Verification items for the finished model (mm, model axes). Give positions to 0.01 mm unless a question says otherwise; leave off trailing zeros. One line per item, written item: value. Start each with the question number.
1. Mould release check, pull along Y, two halves, no side actions. Record for faces 1 (the cylindrical face through (0, 21, 4)), 2 (the cylindrical face through (-36.244, 0.275, 4.437)), 3 (the flat face through (-10, -8, 0)): pulls with the +Y half, pulls with the -Y half, needs draft (parallel to the pull), parting line crosses it, or undercut.
2. Gauge pin test, flat ends, axial feed: pin 1 (5 mm diameter, centred on x = -1.5, z = 2, fed in from +Y); pin 2 (2 mm diameter, centred on y = -7.5, z = 6.5, fed in from +X); pin 3 (4 mm diameter, centred on y = -14.5, z = 3.5, fed in from +X); pin 4 (11 mm diameter, centred on x = -30, y = 0, fed in from +Z). Record the tip position at first contact, or that the pin passes through.
3. Sectioned sample at A-A (y = 2). Count the separate pieces of the cut face and the enclosed holes in it, plus the area to 3 significant figures.
4. Scan lines: L1, parallel to Y at x = 0, z = 6; L2, parallel to Y at x = -30, z = 3.5; L3, parallel to X at y = -3.5, z = 6.75. Record each from-to range of solid material in increasing order. Write a range as [from, to].
from build123d import *

# Parameters (mm, degrees)
F0_R     = 6.25
F0_R_2   = 11
F1_DEPTH = 9
F2_R     = 5
F3_R     = 3
F4_R     = 3


with BuildPart() as f1:
    # F0 (on Top) → F1 (new body)
    with BuildSketch(Plane.XY):
        with BuildLine():
            ThreePointArc((18.965625, 9.0169323142), (20.4850936659, 4.6217894262), (21, 0))
            ThreePointArc((21, 0), (20.4850936659, -4.6217894262), (18.965625, -9.0169323142))
            ThreePointArc((18.965625, -9.0169323142), (34.7865779138, -13.4220405258), (44.25, 0))
            ThreePointArc((44.25, 0), (34.7865779138, 13.4220405258), (18.965625, 9.0169323142))
        make_face()
        with Locations((30, 0)):
            Circle(F0_R, mode=Mode.SUBTRACT)
        with BuildLine():
            ThreePointArc((-15.75, 0), (-16.5779594742, 4.7865779138), (-18.965625, 9.0169323142))
            ThreePointArc((-18.965625, 9.0169323142), (-21, 0), (-18.965625, -9.0169323142))
            ThreePointArc((-18.965625, -9.0169323142), (-16.5779594742, -4.7865779138), (-15.75, 0))
        make_face()
        with BuildLine():
            ThreePointArc((18.965625, -9.0169323142), (20.4850936659, -4.6217894262), (21, 0))
            ThreePointArc((21, 0), (20.4850936659, 4.6217894262), (18.965625, 9.0169323142))
            ThreePointArc((18.965625, 9.0169323142), (15.75, 0), (18.965625, -9.0169323142))
        make_face()
        with BuildLine():
            ThreePointArc((18.965625, -9.0169323142), (15.75, 0), (18.965625, 9.0169323142))
            ThreePointArc((18.965625, 9.0169323142), (0, 21), (-18.965625, 9.0169323142))
            ThreePointArc((-18.965625, 9.0169323142), (-16.5779594742, 4.7865779138), (-15.75, 0))
            ThreePointArc((-15.75, 0), (-16.5779594742, -4.7865779138), (-18.965625, -9.0169323142))
            ThreePointArc((-18.965625, -9.0169323142), (0, -21), (18.965625, -9.0169323142))
        make_face()
        Circle(F0_R_2, mode=Mode.SUBTRACT)
        with BuildLine():
            ThreePointArc((-18.965625, -9.0169323142), (-21, 0), (-18.965625, 9.0169323142))
            ThreePointArc((-18.965625, 9.0169323142), (-44.25, 0), (-18.965625, -9.0169323142))
        make_face()
        with Locations((-30, 0)):
            Circle(F0_R, mode=Mode.SUBTRACT)
    extrude(amount=F1_DEPTH)

    # F2
    f2_edges = [f1.edges().sort_by_distance(p)[0] for p in [
        (-18.965625, 9.016932, 4.5),
        (18.965625, 9.016932, 4.5),
        (-18.965625, -9.016932, 4.5),
        (18.965625, -9.016932, 4.5),
    ]]
    fillet(f2_edges, radius=F2_R)

    # F3
    f3_edges = [f1.edges().sort_by_distance(p)[0] for p in [
        (-44.25, 0, 9),
        (-19.238882, 11.576619, 9),
        (0, 21, 9),
        (19.238882, 11.576619, 9),
        (44.25, 0, 9),
        (19.238882, -11.576619, 9),
        (0, -21, 9),
        (-19.238882, -11.576619, 9),
    ]]
    fillet(f3_edges, radius=F3_R)

    # F4
    f4_edges = [f1.edges().sort_by_distance(p)[0] for p in [
        (-19.238882, -11.576619, 0),
        (-44.25, 0, 0),
        (-19.238882, 11.576619, 0),
        (0, 21, 0),
        (19.238882, 11.576619, 0),
        (44.25, 0, 0),
        (0, -21, 0),
        (19.238882, -11.576619, 0),
    ]]
    fillet(f4_edges, radius=F4_R)


solid = f1.part
Results are:
1. face 1: pulls with the +Y half
1. face 2: undercut
1. face 3: needs draft
2. pin 1: stops at y = 21
2. pin 2: stops at x = 42.65
2. pin 3: stops at x = 36.84
2. pin 4: passes through
3. separate pieces: 4
3. enclosed holes: 0
3. area: 378 mm^2
4. L1: y = [-21, -11], [11, 21]
4. L2: y = [-14.25, -6.25], [6.25, 14.25]
4. L3: x = [-43.72, -35.18], [-24.82, -10.43], [10.43, 24.82], [35.18, 43.72]
